Check sheet for the modelled part. Datum: model origin and axes. Units: mm. A direction names the side the tool comes from. Round coordinates to 2 decimals unless told otherwise and drop trailing zeros. Answer in a Markdown table with one row per item.
```python
from build123d import *

# Parameters (mm, degrees)
EXTRUDE_1_DEPTH     = 150
SKETCH_2_R          = 1.5
CUT_EXTRUDE_1_DEPTH = 6
CUT_EXTRUDE_3_REACH = 302
SKETCH_4_W          = 5
SKETCH_4_H          = 1.5


with BuildPart() as part:
    # 草图1 → 凸台-拉伸1 (new body, symmetric)
    with BuildSketch(Plane.XY):
        Polygon((13, 6), (7.5, 6), (7.5, 4), (4, 4), (4, 2), (6, 0), (-6, 0), (-4, 2), (-4, 4), (-7.5, 4), (-7.5, 6), (-13, 6), (-13, 9), (-8.5, 9), (-8.5, 11), (-5.75, 11), (-5.75, 9.8), (-7.25, 9.8), (-7.25, 8.7), (-5.05, 8.7), (-5.05, 8.2), (5.05, 8.2), (5.05, 8.7), (7.25, 8.7), (7.25, 9.8), (5.75, 9.8), (5.75, 11), (8.5, 11), (8.5, 9), (13, 9), align=None)
    extrude(amount=EXTRUDE_1_DEPTH, both=True)

    # 草图2 → 切除-拉伸1 (cut)
    with BuildSketch(Plane(origin=(0, 0, -150), x_dir=(-1, 0, 0), z_dir=(0, 0, -1))):
        with Locations((0, 5)):
            Circle(SKETCH_2_R)
    cut_extrude_1 = extrude(amount=-CUT_EXTRUDE_1_DEPTH, mode=Mode.SUBTRACT)

    # 草图4 → 切除-拉伸3 (cut, up to next)
    with BuildSketch(Plane.XY.offset(150), mode=Mode.PRIVATE) as cut_extrude_3_sk1:
        with Locations((0, 0.75)):
            Rectangle(SKETCH_4_W, SKETCH_4_H)
    cut_extrude_3_tool1 = extrude(cut_extrude_3_sk1.sketch, amount=-CUT_EXTRUDE_3_REACH, mode=Mode.PRIVATE) & part.part
    add(cut_extrude_3_tool1.solids().sort_by_distance((0, 0.75, 150))[0], mode=Mode.SUBTRACT)

    # 镜向1: 切除-拉伸1 across plane
    add(cut_extrude_1.mirror(Plane.XY), mode=Mode.SUBTRACT)


solid = part.part
```
1. Access from +Z, -Z, +X, -X, +Y, -Y to the whole of each face (thin tool, end or side, straight path). Record for faces 1 (the face through (0, 1.5, 2)), 2 (the face through (10, 6, 2)), 3 (the face through (0, 7, 150)).
Found:
| item | result |
|---|---|
| face 1 | +Z, -Z, -Y |
| face 2 | +Z, -Z, +X, -Y |
| face 3 | +Z, +X, -X, +Y, -Y |
2. Draft check along X on faces 4 (the face through (0, 8.2, 2)), 5 (the face through (-10, 6, 2)). Enter one of: +X half, -X half, draft (parallel to the pull), parting line (faces both ways), or undercut.
Found:
| item | result |
|---|---|
| face 4 | undercut |
| face 5 | draft |
3. Scan lines: L1, parallel to Y at x = 0, z = 146.25; L2, parallel to X at y = 4.5, z = 104; L3, parallel to Y at x = 3.5, z = 88.5. Record each from-to range of solid material in increasing order.
Found:
| item | result |
|---|---|
| L1 | y = 1.5 to 3.5, 6.5 to 8.2 |
| L2 | x = -7.5 to 7.5 |
| L3 | y = 0 to 8.2 |
4. Go/stop test with flat-tipped pins: pin 1 (5 mm diameter, centred on x = 1.5, z = -70.5, fed in from +Y); pin 2 (0.8 mm diameter, centred on y = 0.5, z = 10.5, fed in from -X); pin 3 (2 mm diameter, centred on y = 4, z = -63, fed in from -X). Record where each tip stops, or that it passes through.
Found:
| item | result |
|---|---|
| pin 1 | stops at y = 8.2 |
| pin 2 | stops at x = -5.9 |
| pin 3 | stops at x = -7.5 |
